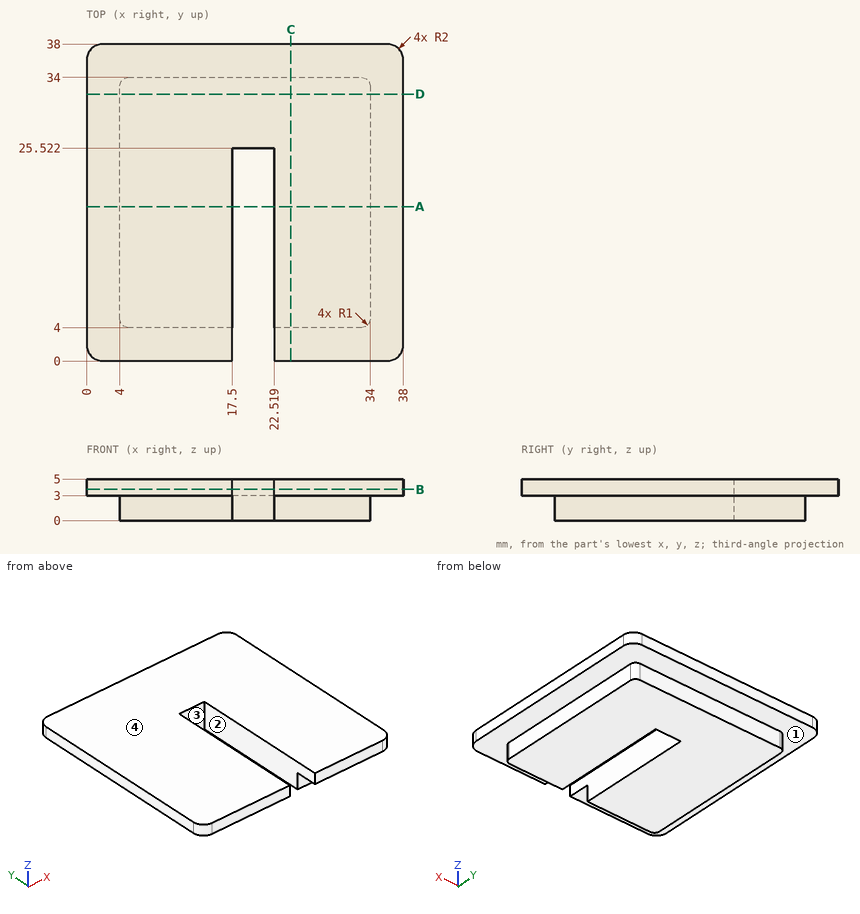
Study the drawing (mm; zero at the part's minimum x, y, z) and answer. A direction names the side the tool comes from. Give positions to 0.01 mm unless a question says otherwise; leave off trailing zeros. Write each loop counter-clockwise with the first axis right and the second up, starting at its lowest first coordinate (ties: lowest second). Pieces come first, ordered by that corner, then holes.
Item 1: Section B-B, the plane z = 3.75 is taken. Write down the section's boundary in (x, y).
Item 2: Find the intervals of material crossed by line 1 along X through (y, z) = (9, 2.2); line 2 along X through (y, z) = (13, 3.85); line 3 along Y through (x, z) = (19.5, 3.55), in increasing order.
Item 3: Section A-A, the plane y = 18.5 is taken. Write down the section's boundary in (x, z).
Item 4: Flat-ended cylindrical pins translate along their axes: P1, Ø1.5, axis at x = 25, z = 1.5, coming from the -Y side; P2, Ø2.5, axis at x = 24.5, z = 1.5, coming from the +Y side; P3, Ø0.9, axis at y = 12.5, z = 2, coming from the -X side; P4, Ø1.5, axis at y = 6.5, z = 2.5, coming from the +X side. Find the tip coordinate at first contact, or state that the pin passes through.
Item 5: Which of the six approach directions +Z, -Z, +X, -X, +Y, -Y give full straight-line access (tool end or side, diameter ignored) to the marked faces 3 and 4?
Item 6: Section C-C, the plane x = 24.5 is taken. Write down the section's boundary in (y, z), plus the area to 3 significant figures.
Item 7: Determine the mould class of the marked faces 1 and 2 for opening direction X: released by +X, released by -X, zero draft, split by the parting line, or undercut.
Completed:
1. outline: (0, 2) arc R2 ccw to (2, 0) - (17.5, 0) - (17.5, 25.52) - (22.52, 25.52) - (22.52, 0) - (36, 0) arc R2 ccw to (38, 2) - (38, 36) arc R2 ccw to (36, 38) - (2, 38) arc R2 ccw to (0, 36) - close
2. line 1: x = 4 to 17.5, 22.52 to 34
2. line 2: x = 0 to 17.5, 22.52 to 38
2. line 3: y = 25.52 to 38
3. outline: (0, 3) - (4, 3) - (4, 0) - (17.5, 0) - (17.5, 5) - (0, 5) - close; (22.52, 0) - (34, 0) - (34, 3) - (38, 3) - (38, 5) - (22.52, 5) - close
4. P1: stops at y = 4
4. P2: stops at y = 34
4. P3: stops at x = 4
4. P4: stops at x = 38
5. face 3: +Z, -Z, -Y
5. face 4: +Z, +X, -X, +Y, -Y
6. outline: (0, 3) - (4, 3) - (4, 0) - (34, 0) - (34, 3) - (38, 3) - (38, 5) - (0, 5) - close
6. area: 166 mm2
7. face 1: zero draft
7. face 2: undercut
